Model file for the job. Use its own axes, mm. Coordinates: 2 decimals unless noted, no trailing zeros. Order: outer loops, then holes, each group sorted by start corner. A loop starts at its lowest first (then second) coordinate and runs counter-clockwise, first axis right, second up. Notation, with made-up numbers: (-10.75, 33.5) -> (48.25, 33.5) arc R24 ccw to (48.25, 57.5) -> close; hole circle Ø10 at (17.25, -23.75). An arc over 180 degrees is marked (long way). Write item = value, one per line. Start each with the question number.
Q1. Flat gauge pins, fed straight in: pin 1 (1.9 mm diameter, centred on y = 339.5, z = -1.5, fed in from -X); pin 2 (2 mm diameter, centred on x = 182, z = -1, fed in from -Y). Where does each tip first touch, or does it go through?
Q2. Cut at C-C, the plane x = 206. List the corners of the cut face in (y, z) (3 decimals).
Q3. Cut at B-B, the plane x = 25.4. List the corners of the cut face in (y, z) (1 decimal), plus the area to 3 significant figures.
Q4. Cut at D-D, the plane y = 96. List the corners of the cut face in (x, z) (3 decimals).
Q5. Cut at A-A, the plane z = 1.5. List the corners of the cut face in (x, y) (1 decimal), plus the area to 3 significant figures.
Q6. Wall check: line 1 (Y direction, x = 162, z = -0.5); line 2 (Y direction, x = 164.5, z = 1.75); line 3 (X direction, y = 253.5, z = 0.25). Give the ranges that are in metal, low to high. Write a range as from..to.
from build123d import *

# Parameters (mm, degrees)
SKETCH1_R           = 14.2875
BOSS_EXTRUDE1_DEPTH = 3.175


with BuildPart() as part:
    # Sketch1 → Boss-Extrude1 (new body, symmetric)
    with BuildSketch(Plane.XY):
        with BuildLine():
            Line((-56.421183023, 233.069398752), (177.06916324, 37.147735319))
            Line((177.06916324, 37.147735319), (258.70318967, 134.435379595))
            Line((258.70318967, 134.435379595), (161.415545394, 216.069406025))
            Line((161.415545394, 216.069406025), (177.74235068, 235.526934881))
            ThreePointArc((177.74235068, 235.526934881), (174.611627111, 271.311269022), (138.82729297, 268.180545453))
            Line((138.82729297, 268.180545453), (122.500487684, 248.723016597))
            Line((122.500487684, 248.723016597), (50.8, 308.886869368))
            Line((50.8, 308.886869368), (50.8, 355.6))
            ThreePointArc((50.8, 355.6), (25.4, 381), (0, 355.6))
            Line((0, 355.6), (0, 300.309546317))
            Line((0, 300.309546317), (-56.421183023, 233.069398752))
        make_face()
        with Locations((25.4, 355.6)):
            Circle(SKETCH1_R, mode=Mode.SUBTRACT)
        with Locations((158.284821825, 251.853740167)):
            Circle(SKETCH1_R, mode=Mode.SUBTRACT)
    extrude(amount=BOSS_EXTRUDE1_DEPTH, both=True)


solid = part.part
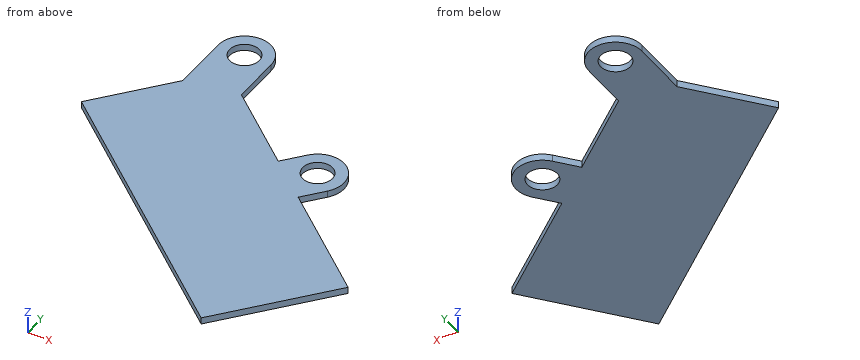
Here are the results:
q1.pin_1 = 0
q1.pin_2 = 41.83
q2.outline = (71.626, -3.175) -> (178.659, -3.175) -> (178.659, 3.175) -> (71.626, 3.175) -> close
q3.outline = (164.4, -3.2) -> (341.3, -3.2) -> (341.3, 3.2) -> (164.4, 3.2) -> close; (369.9, -3.2) -> (381, -3.2) -> (381, 3.2) -> (369.9, 3.2) -> close
q3.area = 1,190 mm²
q4.outline = (106.932, -3.175) -> (226.452, -3.175) -> (226.452, 3.175) -> (106.932, 3.175) -> close
q5.outline = (-56.4, 233.1) -> (177.1, 37.1) -> (258.7, 134.4) -> (161.4, 216.1) -> (177.7, 235.5) arc R25.4 ccw to (138.8, 268.2) -> (122.5, 248.7) -> (50.8, 308.9) -> (50.8, 355.6) arc R25.4 ccw to (0, 355.6) -> (0, 300.3) -> close; hole circle Ø28.6 at (25.4, 355.6); hole circle Ø28.6 at (158.3, 251.9)
q5.area = 42,700 mm²
q6.line_1 = 49.79..215.58, 216.77..238.06, 265.65..276.98
q6.line_2 = 47.69..213.48, 219.75..238.99, 264.72..276.48
q6.line_3 = -39.28..116.81, 126.51..144.09, 172.48..183.63
